Job drawing, mm, ordinate dimensions from the low corner. One solid piece. A direction names the side the tool comes from. Give positions to 0.01 mm unless a question says otherwise; leave off trailing zeros. Write each loop counter-clockwise with the first axis right and the second up, starting at its lowest first coordinate (ties: lowest second). Pieces come first, ordered by that corner, then holes. Notation, with made-up numbers: (57.25, 3) - (88.25, 3) arc R16 ccw to (88.25, 22) - close; hole circle Ø7 at (-5.5, 61.25). An arc over 180 degrees is marked (long way). Put each result on its own line as item: value. Start each with the question number.
1. Mould opens along Z. For the marked faces 1, 2 and 3 say: +Z half, -Z half, draft (parallel to the pull), parting line (faces both ways), or undercut.
2. Tool access for the marked faces 4, 5 and 6: list every direction of +Z, -Z, +X, -X, +Y, -Y with a clear straight run to the whole face (end or side of a thin tool).
3. Wall check: line 1 (Y direction, x = 6.75, z = 4.25); line 2 (Y direction, x = 5.5, z = 5); line 3 (Z direction, x = 4, y = 11.5). Give the ranges that are in metal, low to high.
4. Cut at B-B on z = 2.5. List the corners of the cut face in (x, y).
5. Cut at D-D on x = 7. List the corners of the cut face in (y, z) (1 decimal).
6. Drop flat-ended pins along their axis: pin 1 (4 mm diameter, centred on y = 25.5, z = 5, fed in from -X); pin 2 (0.7 mm diameter, centred on x = 4.5, y = 42, fed in from +Z); pin 3 (1.2 mm diameter, centred on x = 3.5, z = 4.5, fed in from +Y). Give the stop position or say it passes through.
7. Cut at C-C on y = 18.5. List the corners of the cut face in (x, z).
8. Cut at A-A on x = 4. List the corners of the cut face in (y, z), and give its area (3 significant figures).
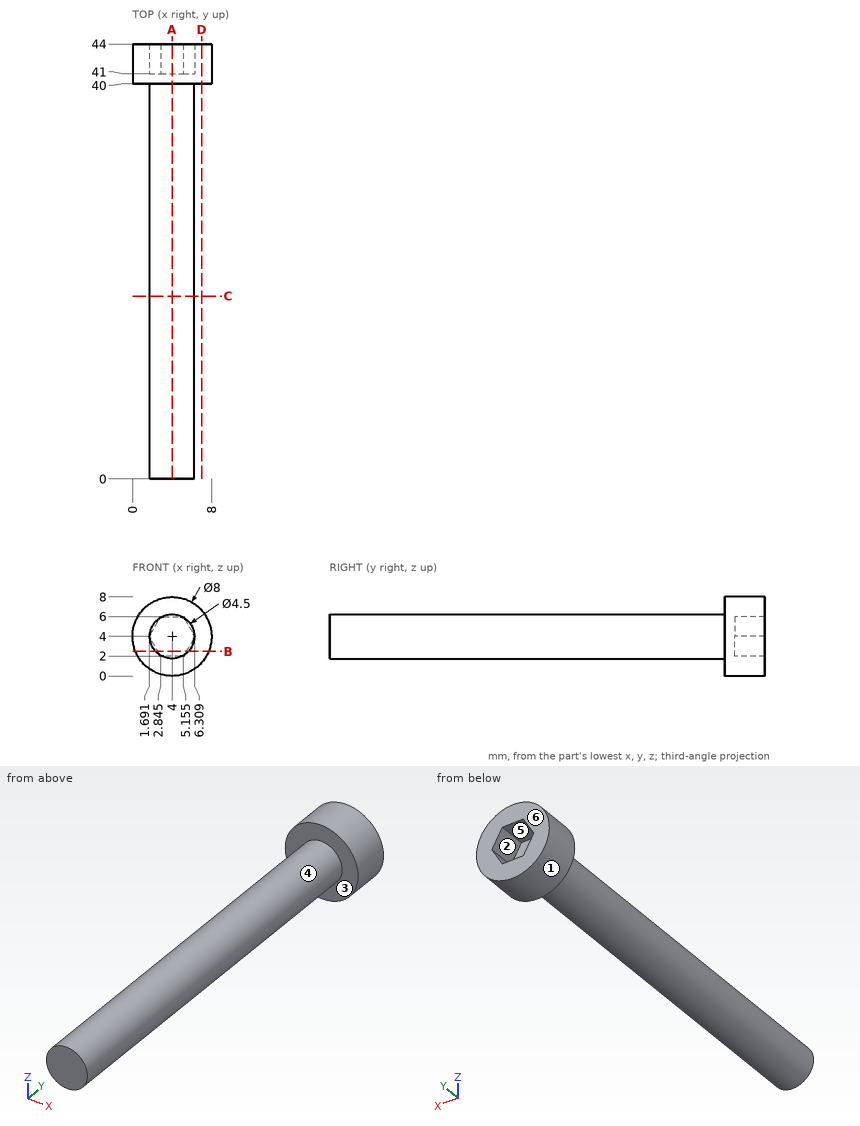
Report:
1. face 1: parting line
1. face 2: undercut
1. face 3: draft
2. face 4: -Y
2. face 5: +Y
2. face 6: +Z, -Z, +X, -X, +Y
3. line 1: y = 40 to 44
3. line 2: y = 0 to 41
3. line 3: z = 1.75 to 6.25
4. outline: (0.29, 40) - (2.32, 40) - (2.32, 0) - (5.68, 0) - (5.68, 40) - (7.71, 40) - (7.71, 44) - (5.44, 44) - (5.44, 41) - (2.56, 41) - (2.56, 44) - (0.29, 44) - close
5. outline: (40, 1.4) - (44, 1.4) - (44, 6.6) - (40, 6.6) - close
6. pin 1: stops at x = 1.75
6. pin 2: stops at z = 8
6. pin 3: stops at y = 41
7. outline: circle Ø4.5 at (4, 4)
8. outline: (0, 1.75) - (40, 1.75) - (40, 0) - (44, 0) - (44, 2) - (41, 2) - (41, 6) - (44, 6) - (44, 8) - (40, 8) - (40, 6.25) - (0, 6.25) - close
8. area: 200 mm²
